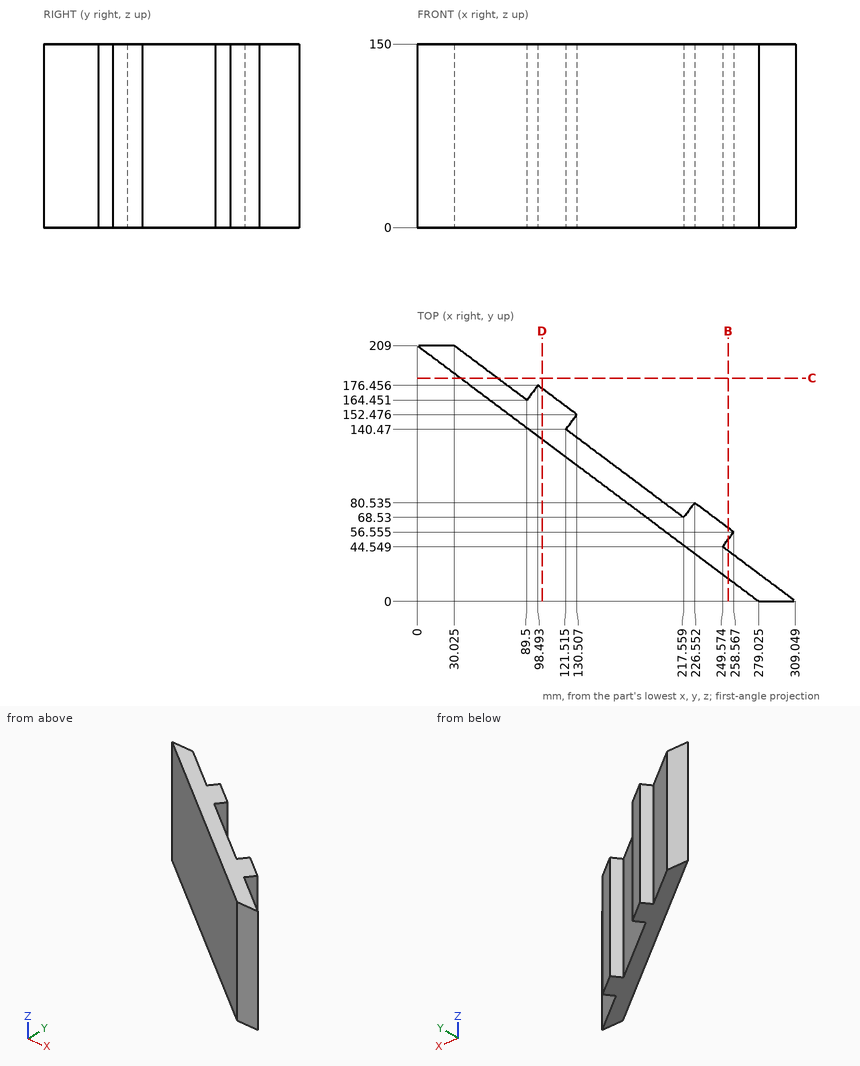
Geometry check sheet. Reference: drawing and pictorial views, mm from the part's lowest x, y, z. Round coordinates to 2 decimals unless told otherwise and drop trailing zeros. Order: outer loops, then holes, each group sorted by start corner. A loop starts at its lowest first (then second) coordinate and runs counter-clockwise, first axis right, second up.
Q1. Depth check by flat-ended pin: P1, Ø1, axis at x = 87.5, z = 41, coming from the -Y side (1 decimal); P2, Ø6, axis at x = 225, z = 63, coming from the -Y side; P3, Ø6, axis at x = 263.5, z = 134, coming from the -Y side. Enter the tip coordinate at first touch or a pass-through.
Filled sheet:
P1: stops at y = 143.1
P2: stops at y = 38.22
P3: stops at y = 9.38
Q2. Scan lines: L1, parallel to X at y = 170.5, z = 57 (1 decimal); L2, parallel to Y at x = 256, z = 96.5 (1 decimal); L3, parallel to X at y = 172, z = 141 (1 decimal). Record each from-to range of solid material in increasing order.
Filled sheet:
L1: x = 51.4 to 81.4, 94 to 106.4
L2: y = 17.2 to 39.7, 53.1 to 58.5
L3: x = 49.4 to 79.4, 95.2 to 104.4
Q3. Cross-section at B-B, the plane x = 254. Enter the section's corners in (y, z) (1 decimal), plus the area to 3 significant figures.
Filled sheet:
outline: (18.7, 0) - (41.2, 0) - (41.2, 150) - (18.7, 150) - close; (50.5, 0) - (60, 0) - (60, 150) - (50.5, 150) - close
area: 4,800 mm2
Q4. Cross-section at C-C, the plane y = 182.5. Enter the section's corners in (x, z), plus the area to 3 significant figures.
Filled sheet:
outline: (35.38, 0) - (65.4, 0) - (65.4, 150) - (35.38, 150) - close
area: 4,500 mm2
Q5. Cross-section at D-D, the plane x = 102. Enter the section's corners in (y, z), plus the area to 3 significant figures.
Filled sheet:
outline: (132.6, 0) - (173.83, 0) - (173.83, 150) - (132.6, 150) - close
area: 6,180 mm2
